from build123d import *

# Parameters (mm, degrees)
SKETCH1_R           = 16.264719519
SKETCH1_R_2         = 1.5
SKETCH1_R_3         = 1.45
BOSS_EXTRUDE1_DEPTH = 2
SKETCH2_R           = 2
CUT_EXTRUDE1_DEPTH  = 119.16416129
FILLET1_R           = 2
SKETCH3_R           = 1
CUT_EXTRUDE2_DEPTH  = 10


with BuildPart() as part:
    # Sketch1 → Boss-Extrude1 (new body)
    with BuildSketch(Plane(origin=(0, 0, 0), x_dir=(1, 0, 0), z_dir=(0, 1, 0))):
        with BuildLine():
            Line((-12.392234006, -6.981301864), (-12.392234006, -30.758658484))
            Line((-12.392234006, -30.758658484), (-12.392234006, -37.869980174))
            Line((-12.392234006, -37.869980174), (-12.392234006, -39.662475092))
            ThreePointArc((-12.392234006, -39.662475092), (-11.513554349, -41.783795436), (-9.392234006, -42.662475092))
            Line((-9.392234006, -42.662475092), (8.128346254, -42.662475092))
            Line((8.128346254, -42.662475092), (8.128346254, -49.872480174))
            Line((8.128346254, -49.872480174), (-11.871653746, -69.872480174))
            Line((-11.871653746, -69.872480174), (-49.281653746, -69.872480174))
            Line((-49.281653746, -69.872480174), (-61.796944846, -53.596788721))
            Line((-61.796944846, -53.596788721), (-74.058017443, -53.596788721))
            Line((-74.058017443, -53.596788721), (-95.271220878, -38.596788721))
            Line((-95.271220878, -38.596788721), (-95.271220878, -26.897908721))
            Line((-95.271220878, -26.897908721), (-84.130114655, -26.897908721))
            Line((-84.130114655, -26.897908721), (-83.276622696, -26.897908721))
            Line((-83.276622696, -26.897908721), (-83.276622696, 11.130019826))
            Line((-83.276622696, 11.130019826), (-60.448477034, 11.130019826))
            Line((-60.448477034, 11.130019826), (-49.281653746, 32.132519826))
            Line((-49.281653746, 32.132519826), (-11.871653746, 32.132519826))
            Line((-11.871653746, 32.132519826), (8.128346254, 12.132519826))
            Line((8.128346254, 12.132519826), (8.128346254, 4.922514744))
            Line((8.128346254, 4.922514744), (-9.392234006, 4.922514744))
            ThreePointArc((-9.392234006, 4.922514744), (-11.513554349, 4.043835088), (-12.392234006, 1.922514744))
            Line((-12.392234006, 1.922514744), (-12.392234006, 0.130019826))
            Line((-12.392234006, 0.130019826), (-12.392234006, -6.981301864))
        make_face()
        with Locations(Location((-37.781653746, -48.747480173, 0), (0, 0, 270))):
            Circle(SKETCH1_R, mode=Mode.SUBTRACT)
        with Locations(Location((-37.781653746, 11.007519825, 0), (0, 0, 90))):
            Circle(SKETCH1_R, mode=Mode.SUBTRACT)
        with Locations(Location((-15.087114055, -5.127161907, 0), (0, 0, 270))):
            Circle(SKETCH1_R_2, mode=Mode.SUBTRACT)
        with Locations(Location((-15.087114055, -32.612798441, 0), (0, 0, 270))):
            Circle(SKETCH1_R_2, mode=Mode.SUBTRACT)
        with Locations(Location((-81.12792954, -12.064242343, 0), (0, 0, 270))):
            Circle(SKETCH1_R_3, mode=Mode.SUBTRACT)
        with Locations(Location((-75.470082252, -19.063439731, 0), (0, 0, 270))):
            Circle(SKETCH1_R_3, mode=Mode.SUBTRACT)
        with Locations(Location((-68.470884865, -24.721287018, 0), (0, 0, 270))):
            Circle(SKETCH1_R_3, mode=Mode.SUBTRACT)
        with Locations(Location((-92.311157954, -34.437864429, 0), (0, 0, 270))):
            Circle(SKETCH1_R_2, mode=Mode.SUBTRACT)
        with Locations(Location((-66.462987255, -49.872480174, 0), (0, 0, 270))):
            Circle(SKETCH1_R_2, mode=Mode.SUBTRACT)
        with Locations(Location((-80.455556672, 8.666951386, 0), (0, 0, 270))):
            Circle(SKETCH1_R_2, mode=Mode.SUBTRACT)
        with BuildLine():
            Line((-52.664953624, -16.00672876), (-53.702548501, -19.879085561))
            ThreePointArc((-53.702548501, -19.879085561), (-54.689042095, -21.123916801), (-56.271766971, -21.257169903))
            ThreePointArc((-56.271766971, -21.257169903), (-69.478161637, -13.071519115), (-77.663812425, 0.13487555))
            ThreePointArc((-77.663812425, 0.13487555), (-77.530559323, 1.717600427), (-76.285728083, 2.70409402))
            Line((-76.285728083, 2.70409402), (-72.413371282, 3.741688898))
            ThreePointArc((-72.413371282, 3.741688898), (-70.958270463, 3.576518776), (-70.005790184, 2.464142545))
            ThreePointArc((-70.005790184, 2.464142545), (-63.821307387, -7.414664865), (-53.942499976, -13.599147662))
            ThreePointArc((-53.942499976, -13.599147662), (-52.830123745, -14.551627941), (-52.664953624, -16.00672876))
        make_face(mode=Mode.SUBTRACT)
    extrude(amount=BOSS_EXTRUDE1_DEPTH)

    # Sketch2 → Cut-Extrude1 (cut, through all)
    with BuildSketch(Plane(origin=(0, 2, 0), x_dir=(1, 0, 0), z_dir=(0, 1, 0))):
        with Locations(Location((-13.067528443, -65.799136603, 0), (0, 0, 270))):
            Circle(SKETCH2_R)
        with Locations(Location((-13.067528443, 28.059176255, 0), (0, 0, 270))):
            Circle(SKETCH2_R)
    extrude(amount=-CUT_EXTRUDE1_DEPTH, mode=Mode.SUBTRACT)

    # Fillet1
    fillet1_edges = [part.edges().sort_by_distance(p)[0] for p in [
        (-49.281653746, 1, -32.132519826),
        (-11.871653746, 1, -32.132519826),
        (8.128346254, 1, -12.132519826),
        (8.128346254, 1, -4.922514744),
        (8.128346254, 1, 42.662475092),
        (8.128346254, 1, 49.872480174),
        (-11.871653746, 1, 69.872480174),
        (-49.281653746, 1, 69.872480174),
        (-61.796944846, 1, 53.596788721),
        (-74.058017443, 1, 53.596788721),
        (-95.271220878, 1, 38.596788721),
        (-95.271220878, 1, 26.897908721),
        (-83.276622696, 1, -11.130019826),
        (-60.448477034, 1, -11.130019826),
    ]]
    fillet(fillet1_edges, radius=FILLET1_R)

    # Sketch3 → Cut-Extrude2 (cut)
    with BuildSketch(Plane(origin=(0, 2, 0), x_dir=(1, 0, 0), z_dir=(0, 1, 0))):
        with Locations((-83.276622696, -26.897908721)):
            Circle(SKETCH3_R)
    extrude(amount=-CUT_EXTRUDE2_DEPTH, mode=Mode.SUBTRACT)


solid = part.part
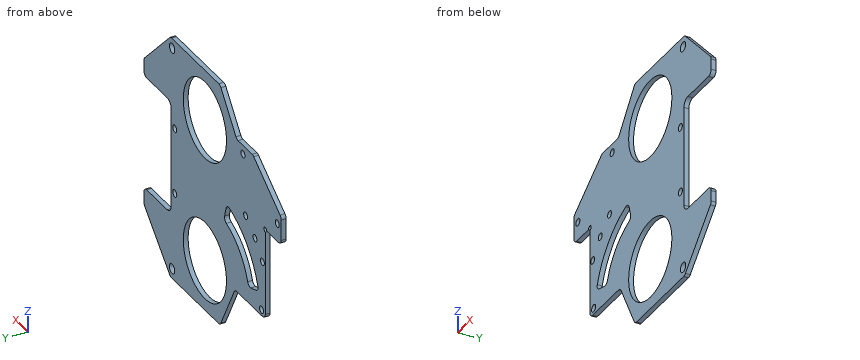
Verification items for the finished model (mm, model axes). Coordinates: 2 decimals unless noted, no trailing zeros. Write each loop counter-clockwise with the first axis right and the second up, starting at its lowest first coordinate (ties: lowest second). Pieces come first, ordered by that corner, then holes. Notation, with made-up numbers: (-3, -34) - (38, -34) arc R28 ccw to (38, 4) - close; hole circle Ø7 at (16, -32.75). An arc over 180 degrees is marked (long way). Answer as a JSON object with one key per item and string values.
(1) Gauge pin test, flat ends, axial feed: pin 1 Ø1 at (x, y) = (-71, 1) entering from -Z; pin 2 Ø1 at (y, z) = (0.5, -9.5) entering from -X; pin 3 Ø1 at (x, y) = (-85, 0) entering from -Z. Record the tip position at first contact, or that the pin passes through.
Report:
{"pin 1": "z = -11.13", "pin 2": "x = -83.28", "pin 3": "z = 26.9"}
(2) Cross-section at C-C on x = 1.5. Record the cut outline in (y, z).
Report:
{"outline": "(0, -18.76) - (2, -18.76) - (2, -4.92) - (0, -4.92) - close; (0, 42.66) - (2, 42.66) - (2, 56.5) - (0, 56.5) - close"}
(3) Thickness scan on line 1 along Z through (x, y) = (-65.5, 0.85); line 2 along Z through (x, y) = (-48, 0.35); line 3 along X through (y, z) = (1.55, -8). Record the ranges inside material, lowest first.
Report:
{"line 1": "-11.13 to 5.57, 16.48 to 48.72, 51.02 to 53.6", "line 2": "-32.13 to -23.66, 1.65 to 36.09, 61.4 to 69.87", "line 3": "-83.28 to -81.8, -79.11 to -53.77, -21.8 to 8.13"}
(4) Cross-section at D-D on y = 1.15. Give the number of separate pieces and of enclosed holes in the cut face, plus the area to 3 significant figures.
Report:
{"separate pieces": "1", "enclosed holes": "13", "area": "5,070 mm^2"}
(5) Cross-section at B-B on z = -14.5. Record the cut outline in (x, y), plus the area to 3 significant figures.
Report:
{"outline": "(-58.66, 0) - (-53.67, 0) - (-53.67, 2) - (-58.66, 2) - close; (-21.9, 0) - (5.76, 0) - (5.76, 2) - (-21.9, 2) - close", "area": "65.3 mm^2"}
(6) Cross-section at A-A on x = -39. Record the cut outline in (y, z).
Report:
{"outline": "(0, -32.13) - (2, -32.13) - (2, -27.23) - (0, -27.23) - close; (0, 5.21) - (2, 5.21) - (2, 32.53) - (0, 32.53) - close; (0, 64.97) - (2, 64.97) - (2, 69.87) - (0, 69.87) - close"}
